Geometry check sheet. Reference: the model listing, model coordinates, mm. A direction names the side the tool comes from. Give positions to 0.01 mm unless a question says otherwise; leave off trailing zeros. Write each loop counter-clockwise with the first axis right and the second up, starting at its lowest first coordinate (ties: lowest second). Pieces come first, ordered by that corner, then holes. Notation, with made-up numbers: (-32, -15.5) -> (-22, -15.5) arc R16 cw to (-22, 5.5) -> close; hole circle Ø7 at (64, -24). An arc over 180 degrees is marked (long way). One line per item, written item: value.
from build123d import *

# Parameters (mm, degrees)
CHAMFER1_SIZE = 0.5


with BuildPart() as part:
    # Sketch1 → Revolve1 (revolve)
    with BuildSketch(Plane(origin=(0, 0, 0), x_dir=(1, 0, 0), z_dir=(0, 1, 0))):
        Polygon((0, 27.73647874), (4.15, 27.73647874), (4.15, 37.73647874), (50, 37.73647874), (50, -12.26352126), (14.15, -62.26352126), (8.15, -62.26352126), (8.15, -12.26352126), (0, -12.26352126), align=None)
    revolve(axis=Axis((0, 0, 12.26352126), (0, 0, -1)))

    # Chamfer1
    chamfer1_edges = [part.edges().sort_by_distance(p)[0] for p in [
        (-8.15, 0, 62.26352126),
        (-50, 0, -37.73647874),
        (-4.15, 0, -37.73647874),
    ]]
    chamfer(chamfer1_edges, length=CHAMFER1_SIZE)


solid = part.part
1) Tool access check on faces 5 (the cylindrical face through (47.69, -15.02, -12.14)), 6 (the flat face through (0, 0, -27.736)), 7 (the flat face through (0, 0, 12.264)). Record the directions out of +Z, -Z, +X, -X, +Y, -Y that give a thin tool (end or side, any length) a straight path to the whole face; none if there is none.
Verdict:
face 5: +Z, -Z
face 6: -Z
face 7: +Z
2) Sectioned sample at C-C on z = -5.5. Record the cut outline in (x, y).
Verdict:
outline: circle Ø100 at (0, 0)
3) Depth check by flat-ended pin: pin 1 Ø4 at (x, z) = (13, 48) entering from +Y; pin 2 Ø6 at (x, y) = (-14, 11.5) entering from +Z; pin 3 Ø6.5 at (x, y) = (0, 0) entering from -Z. Enter the tip coordinate at first touch or a pass-through.
Verdict:
pin 1: y = 22.64
pin 2: z = 60.91
pin 3: z = -27.74
4) Mould release check, pull along X, two halves, no side actions. Record for faces 1 (the cylindrical face through (-6.468, 4.959, 36.667)), 2 (the flat face through (-6.5, 6.1, 62.264)), 3 (the conical face through (-15.771, 12.093, 54.28)), 4 (the cylindrical face through (-0.9, 4.05, -32.55)): released by +X, released by -X, zero draft, split by the parting line, or undercut.
Verdict:
face 1: undercut
face 2: zero draft
face 3: split by the parting line
face 4: undercut
5) Scan lines: probe 1 along Y at (x, z) = (0, -32); probe 2 along Y at (x, z) = (-3, 36). Record each from-to range of solid material in increasing order.
Verdict:
probe 1: -50 to -4.15, 4.15 to 50
probe 2: -32.84 to -7.58, 7.58 to 32.84
6) Sectioned sample at A-A on y = 0. Record the cut outline in (x, z), plus the area to 3 significant figures.
Verdict:
outline: (-50, -37.24) -> (-49.5, -37.74) -> (-4.65, -37.74) -> (-4.15, -37.24) -> (-4.15, -27.74) -> (4.15, -27.74) -> (4.15, -37.24) -> (4.65, -37.74) -> (49.5, -37.74) -> (50, -37.24) -> (50, 12.26) -> (14.15, 62.26) -> (8.65, 62.26) -> (8.15, 61.76) -> (8.15, 12.26) -> (-8.15, 12.26) -> (-8.15, 61.76) -> (-8.65, 62.26) -> (-14.15, 62.26) -> (-50, 12.26) -> close
area: 7,310 mm^2
7) Sectioned sample at D-D on z = 29.5. Record the cut outline in (x, y).
Verdict:
outline: circle Ø75.28 at (0, 0); hole circle Ø16.3 at (0, 0)
